The model under review builds one solid part; all positions refer to its coordinate system, in mm. Coordinates: 2 decimals unless noted, no trailing zeros. Write each loop counter-clockwise with the first axis right and the second up, starting at its lowest first coordinate (ties: lowest second). Pieces come first, ordered by that corner, then holes. Notation, with made-up numbers: M -14.75,35.5 L 27.25,35.5 A21 cw 27.25,65.5 Z; hole C 77,-20.5 d2. An arc over 180 degrees is marked long. Answer as a JSON object with one key per item and string values.
Autodesk Inventor part; units mm, degrees
ref_plane "YZ Plane" through (0, 0, 0) normal (1, 0, 0) x (0, 1, 0)
ref_plane "XZ Plane" through (0, 0, 0) normal (0, 1, 0) x (-1, 0, 0)
ref_plane "XY Plane" through (0, 0, 0) normal (0, 0, 1) x (1, 0, 0)
sketch "Sketch1" plane through (0, 0, 0) normal (0, 1, 0) x (-1, 0, 0)
  circle A0 centre (0, 0) radius 2.75
  line L0 (2.75, -1.5877) -> (0, -3.1754)
  line L1 (0, -3.1754) -> (-2.75, -1.5877)
  line L2 (-2.75, -1.5877) -> (-2.75, 1.5877)
  line L3 (-2.75, 1.5877) -> (0, 3.1754)
  line L4 (0, 3.1754) -> (2.75, 1.5877)
  line L5 (2.75, 1.5877) -> (2.75, -1.5877)
  circle A1 centre (0, 0) radius 1.25
  point P0 (2.75, 0)
  dimension "d0" = 5.5
  dimension "d1" = 2.5
extrude "Extrusion1" add sketch "Sketch1" along normal blind 30
thread "Thread1"
sketch "Sketch2" plane through (0, 30, 0) normal (0, 1, 0) x (1, 0, 0)
  line L0 (-7.5964, -8.221) -> (7.9188, -8.221)
  line L1 (7.9188, -8.221) -> (7.9188, 5.8837)
  line L2 (7.9188, 5.8837) -> (-7.5964, 5.8837)
  line L3 (-7.5964, 5.8837) -> (-7.5964, -8.221)
  point P0 (0, 0)
extrude "Extrusion2" cut sketch "Sketch2" against normal blind 10
properties part number "Distance_M3_20" material "Nickel-Copper Alloy 400"
(1) Wall thickness on line 1 along X through (y, z) = (19, 0); line 2 along X through (y, z) = (7.5, -0.5); line 3 along Z through (x, y) = (0.05, 6.5): over which ranges is each line inside the solid? List them lowest first. Write a range as from..to.
Results list:
{"line 1": "-2.75..-1.25, 1.25..2.75", "line 2": "-2.75..-1.15, 1.15..2.75", "line 3": "-3.15..-1.25, 1.25..3.15"}
(2) Draft analysis for pull direction Z (two halves, no side actions). For faces 1 (the face through (-1.36, 9.86, 2.39)), 2 (the face through (1.36, 9.86, -2.39)), 3 (the face through (-2.75, 10, 0)), 4 (the face through (0.27, 9.86, 1.22)), state which applies: released by +Z, released by -Z, zero draft, split by the parting line, or undercut.
Results list:
{"face 1": "released by +Z", "face 2": "released by -Z", "face 3": "zero draft", "face 4": "undercut"}
(3) Add section C-C on x = -0.55. Give the boundary of the cut face in (y, z), and give its area (3 significant figures).
Results list:
{"outline": "M 0,-2.86 L 20,-2.86 L 20,-1.12 L 0,-1.12 Z; M 0,1.12 L 20,1.12 L 20,2.86 L 0,2.86 Z", "area": "69.4 mm²"}
(4) For pin 1 Ø3 at (y, z) = (4, -2) entering from -X, flat-tipped, find the tip position at first contact; note if it passes through.
Results list:
{"pin 1": "x = -2.75"}
(5) Add section A-A on z = 0. Give the boundary of the cut face in (x, y).
Results list:
{"outline": "M -2.75,0 L -1.25,0 L -1.25,20 L -2.75,20 Z; M 1.25,0 L 2.75,0 L 2.75,20 L 1.25,20 Z"}
(6) Add section B-B on y = 18.75. Give the boundary of the cut face in (x, z), and give its area (3 significant figures).
Results list:
{"outline": "M -2.75,-1.59 L 0,-3.18 L 2.75,-1.59 L 2.75,1.59 L 0,3.18 L -2.75,1.59 Z; hole C 0,0 d2.5", "area": "21.3 mm²"}
(7) Add section D-D on x = -2.3. Give the boundary of the cut face in (y, z).
Results list:
{"outline": "M 0,-1.85 L 20,-1.85 L 20,1.85 L 0,1.85 Z"}
